Autodesk Fusion 360 part; units mm, degrees
sketch "Sketch1" plane through (0, 0, 0) normal (1, 0, 0) x (0, 1, 0)
  line L0 (0, 0) -> (9.5, 0)
  line L1 (0, 0) -> (0, 8) construction
  line L2 (0, 8) -> (11.5, 8)
  line L3 (11.5, 8) -> (11.5, 4.5)
  line L4 (11.5, 4.5) -> (9.5, 4.5)
  line L5 (9.5, 4.5) -> (9.5, 0)
  line L6 (-9.5, 4.5) -> (-9.5, 0)
  line L7 (-11.5, 8) -> (-11.5, 4.5)
  line L8 (0, 0) -> (-9.5, 0)
  line L9 (0, 8) -> (-11.5, 8)
  line L10 (-11.5, 4.5) -> (-9.5, 4.5)
  dimension "d1" = 9.5
  dimension "d2" = 8
  dimension "d3" = 11.5
  dimension "d4" = 3.5
extrude "Extrude1" add sketch "Sketch1" along normal mid plane 100
sketch "Sketch2" plane through (0, 0, 8) normal (0, 0, 1) x (-1, 0, 0)
  line L0 (50, 11.5) -> (-50, 11.5)
  line L1 (-50, 11.5) -> (-50, -11.5)
  line L2 (-50, -11.5) -> (50, -11.5)
  line L3 (50, -11.5) -> (50, 11.5)
  line L4 (50, 0) -> (40, 0) construction
  circle A0 centre (40, 0) radius 3
  line L5 (40, 0) -> (20, 0) construction
  circle A1 centre (20, 0) radius 4
  dimension "d11" = 10
  dimension "d12" = 6
  dimension "d13" = 20
  dimension "d14" = 8
extrude "Extrude2" cut sketch "Sketch2" against normal up to surface (8 mm away) contours A0 | A1
pattern_linear "R-Pattern1" count 5 spacing 40 along (1, 0, 0) of "Extrude2"
equation "d1 = ( 19 / 2 ) * 1 mm"
equation "d3 = ( 23 / 2 ) * 1 mm"
equation "Alu_M6_M8_T_track_length_slider = 100 mm"
equation "d6 = Alu_M6_M8_T_track_length_slider / 2"
Verification items for the finished model (mm, model axes). A direction names the side the tool comes from. Coordinates: 2 decimals unless noted, no trailing zeros. Order: outer loops, then holes, each group sorted by start corner. A loop starts at its lowest first (then second) coordinate and runs counter-clockwise, first axis right, second up. Notation, with made-up numbers: (50, -9.75) -> (81, -9.75) arc R26 ccw to (81, 19.25) -> close; hole circle Ø4 at (81.25, -11.5). An arc over 180 degrees is marked (long way). Use CSV: the item, a comma, the result in double quotes. Start each with the question number.
Q1. Depth check by flat-ended pin: P1, Ø0.6, axis at x = 14, y = 10.5, coming from the -Z side; P2, Ø2, axis at x = 4, z = 3, coming from the -Y side; P3, Ø1.3, axis at x = 1.5, z = 2, coming from the +Y side. Enter the tip coordinate at first touch or a pass-through.
Q2. Section check B-B, the plane y = 0. Record the cut outline in (x, z).
Q3. Section check C-C, the plane x = 20. Record the cut outline in (y, z), and give its area (3 significant figures).
Q4. Section check A-A, the plane z = 7. Record the cut outline in (x, y).
Q5. Tool access check on faces 1 (the flat face through (-1, 9.5, 2)), 2 (the cylindrical face through (-16.8, 2.4, 4.1)), 3 (the flat face through (-1, -9.5, 2)). Record the directions out of +Z, -Z, +X, -X, +Y, -Y that give a thin tool (end or side, any length) a straight path to the whole face; none if there is none.
Q6. Draft check along X on faces 4 (the flat face through (50, 0, 4)), 5 (the flat face through (-1, 5, 8)), 6 (the cylindrical face through (-37, 0, 4)). Enter one of: +X half, -X half, draft (parallel to the pull), parting line (faces both ways), or undercut.
Q7. Section check D-D, the plane x = -36. Record the cut outline in (y, z).
Q8. Thickness scan on line 1 along X through (y, z) = (0, 4); line 2 along Y through (x, z) = (40, 3.75); line 3 along X through (y, z) = (1.75, 7). Record the ranges inside material, lowest first.
Returned:
1,P1,"stops at z = 4.5"
1,P2,"stops at y = -9.5"
1,P3,"stops at y = 9.5"
2,outline,"(-50, 0) -> (-43, 0) -> (-43, 8) -> (-50, 8) -> close; (-37, 0) -> (-24, 0) -> (-24, 8) -> (-37, 8) -> close; (-16, 0) -> (-3, 0) -> (-3, 8) -> (-16, 8) -> close; (3, 0) -> (16, 0) -> (16, 8) -> (3, 8) -> close; (24, 0) -> (37, 0) -> (37, 8) -> (24, 8) -> close; (43, 0) -> (50, 0) -> (50, 8) -> (43, 8) -> close"
3,outline,"(-11.5, 4.5) -> (-9.5, 4.5) -> (-9.5, 0) -> (-4, 0) -> (-4, 8) -> (-11.5, 8) -> close; (4, 0) -> (9.5, 0) -> (9.5, 4.5) -> (11.5, 4.5) -> (11.5, 8) -> (4, 8) -> close"
3,area,"102 mm^2"
4,outline,"(-50, -11.5) -> (50, -11.5) -> (50, 11.5) -> (-50, 11.5) -> close; hole circle Ø6 at (-40, 0); hole circle Ø8 at (-20, 0); hole circle Ø6 at (0, 0); hole circle Ø8 at (20, 0); hole circle Ø6 at (40, 0)"
5,face 1,"-Z, +X, -X, +Y"
5,face 2,"+Z, -Z"
5,face 3,"-Z, +X, -X, -Y"
6,face 4,"+X half"
6,face 5,"draft"
6,face 6,"undercut"
7,outline,"(-11.5, 4.5) -> (-9.5, 4.5) -> (-9.5, 0) -> (9.5, 0) -> (9.5, 4.5) -> (11.5, 4.5) -> (11.5, 8) -> (-11.5, 8) -> close"
8,line 1,"x = -50 to -43, -37 to -24, -16 to -3, 3 to 16, 24 to 37, 43 to 50"
8,line 2,"y = -9.5 to -3, 3 to 9.5"
8,line 3,"x = -50 to -42.44, -37.56 to -23.6, -16.4 to -2.44, 2.44 to 16.4, 23.6 to 37.56, 42.44 to 50"
